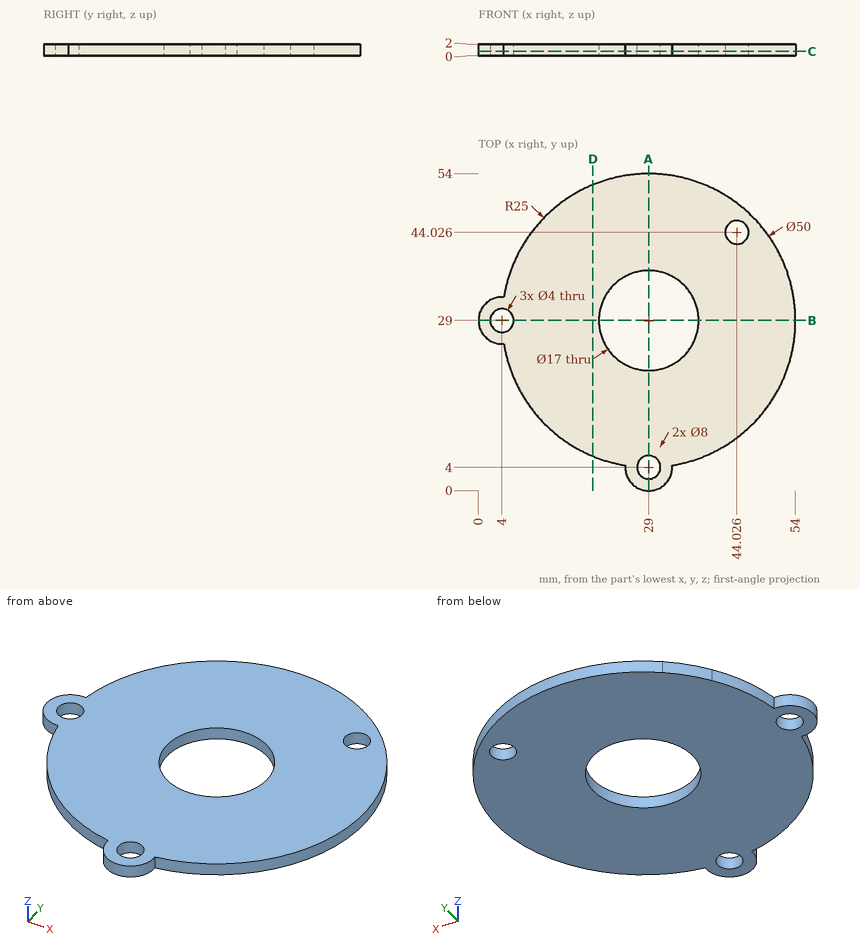
Geometry check sheet. Reference: drawing and pictorial views, mm from the part's lowest x, y, z. Give positions to 0.01 mm unless a question says otherwise; leave off trailing zeros. Write each loop counter-clockwise with the first axis right and the second up, starting at its lowest first coordinate (ties: lowest second). Pieces come first, ordered by that corner, then holes. Notation, with made-up numbers: M -2,20 L 8,20 A26 cw 8,48 Z; hole C 77,-10.75 d7. An arc over 180 degrees is marked long. Put each result on its own line as item: value. Start each with the question number.
1. Section check D-D (x = 19.5). Record the cut outline in (y, z).
2. Go/stop test with flat-tipped pins: pin 1 Ø6 at (x, y) = (47, 7.5) entering from +Z; pin 2 Ø1 at (y, z) = (40.5, 1.5) entering from +X; pin 3 Ø1 at (y, z) = (6, 0.5) entering from +X; pin 4 Ø6.5 at (x, y) = (44.03, 44.03) entering from +Z. Record where each tip stops, or that it passes through.
3. Section check A-A (x = 29). Record the cut outline in (y, z).
4. Section check C-C (z = 0.75). Record the cut outline in (x, y).
5. Scan lines: line 1 along Y through (x, z) = (29, 0.65); line 2 along X through (y, z) = (28, 1.05); line 3 along Y through (x, z) = (4, 1.3). Record each from-to range of solid material in increasing order. Write a range as [from, to].
Answer list:
1. outline: M 5.88,0 L 52.12,0 L 52.12,2 L 5.88,2 Z
2. pin 1: through
2. pin 2: x = 51.45
2. pin 3: x = 39.9
2. pin 4: z = 2
3. outline: M 0,0 L 2,0 L 2,2 L 0,2 Z; M 6,0 L 20.5,0 L 20.5,2 L 6,2 Z; M 37.5,0 L 54,0 L 54,2 L 37.5,2 Z
4. outline: M 4.32,25.01 A25 ccw 25.01,4.32 A4 ccw long 32.99,4.32 A25 ccw long 4.32,32.99 A4 ccw long Z; hole C 4,29 d4; hole C 29,29 d17; hole C 29,4 d4; hole C 44.03,44.03 d4
5. line 1: [0, 2], [6, 20.5], [37.5, 54]
5. line 2: [0.13, 2.27], [5.73, 20.56], [37.44, 53.98]
5. line 3: [25, 27], [31, 33]
